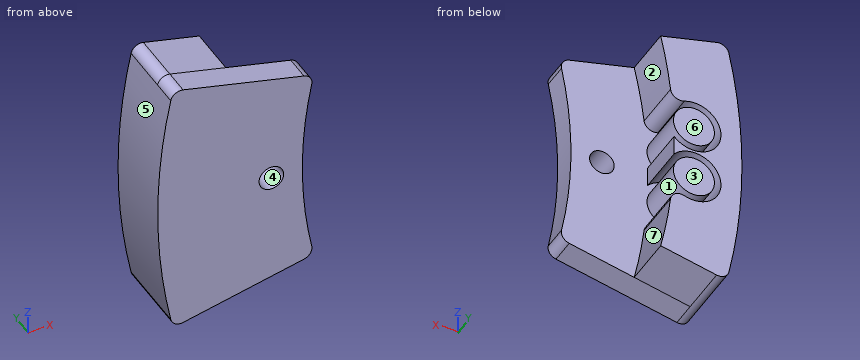
from build123d import *

# Parameters (mm, degrees)
SKETCH2_R           = 2.4
BOSS_EXTRUDE1_DEPTH = 5
BOSS_EXTRUDE2_DEPTH = 10
SKETCH4_R           = 5.27
SKETCH4_R_2         = 4
CUT_EXTRUDE1_DEPTH  = 10
CUT_EXTRUDE2_DEPTH  = 6
FILLET1_R           = 2


with BuildPart() as part:
    # Sketch2 → Boss-Extrude1 (new body)
    with BuildSketch(Plane(origin=(0, 0, 0), x_dir=(1, 0, 0), z_dir=(0, 1, 0))):
        with BuildLine():
            Line((100.252220984, 12.5), (-12.802476078, 38.600733409))
            ThreePointArc((-12.802476078, 38.600733409), (-15.776279016, 12.5), (-12.802476078, -13.600733409))
            Line((-12.802476078, -13.600733409), (100.252220984, 12.5))
        make_face()
        with Locations((6.397320984, 12.5)):
            Circle(SKETCH2_R, mode=Mode.SUBTRACT)
    extrude(amount=BOSS_EXTRUDE1_DEPTH)

    # Sketch3 → Boss-Extrude2 (add)
    with BuildSketch(Plane(origin=(0, 5, 0), x_dir=(1, 0, 0), z_dir=(0, 1, 0))):
        with BuildLine():
            Line((0.080644919, -10.626430568), (-12.802476078, -13.600733409))
            ThreePointArc((-12.802476078, -13.600733409), (-15.776279016, 12.5), (-12.802476078, 38.600733409))
            Line((-12.802476078, 38.600733409), (0.080644919, 35.626430568))
            ThreePointArc((0.080644919, 35.626430568), (-2.554279016, 12.5), (0.080644919, -10.626430568))
        make_face()
    extrude(amount=BOSS_EXTRUDE2_DEPTH)

    # Sketch4 → Cut-Extrude1 (cut)
    with BuildSketch(Plane(origin=(0, 15, 0), x_dir=(1, 0, 0), z_dir=(0, 1, 0))):
        with Locations((-6.412573781, 7)):
            Circle(SKETCH4_R)
        with Locations((-6.412573781, 7)):
            Circle(SKETCH4_R_2, mode=Mode.SUBTRACT)
    cut_extrude1 = extrude(amount=-CUT_EXTRUDE1_DEPTH, mode=Mode.SUBTRACT)

    # Mirror1: Cut-Extrude1 across plane
    add(cut_extrude1.mirror(Plane.XY.offset(-12.5)), mode=Mode.SUBTRACT)

    # Sketch5 → Cut-Extrude2 (cut, through all)
    with BuildSketch(Plane(origin=(0, 5, 0), x_dir=(1, 0, 0), z_dir=(0, 1, 0))):
        with BuildLine():
            Line((14.696195891, -7.252164753), (100.252220984, 12.5))
            Line((100.252220984, 12.5), (14.696195891, 32.252164753))
            ThreePointArc((14.696195891, 32.252164753), (12.445720984, 12.5), (14.696195891, -7.252164753))
        make_face()
    extrude(amount=-CUT_EXTRUDE2_DEPTH, mode=Mode.SUBTRACT)

    # Fillet1
    fillet1_edges = [part.edges().sort_by_distance(p)[0] for p in [
        (-2.189516169, 10, -3.847432094),
        (-2.189516169, 10, -21.152567906),
        (-12.802476078, 7.5, 13.600733409),
        (14.696195891, 2.5, -32.252164753),
        (-12.802476078, 7.5, -38.600733409),
        (14.696195891, 2.5, 7.252164753),
    ]]
    fillet(fillet1_edges, radius=FILLET1_R)


solid = part.part
Source: CAD feature listing. Evaluate the final solid. Frame: model axes, mm. Face numbers are marked on the shaded views. A direction names the side the tool comes from. Give positions to 0.01 mm unless a question says otherwise; leave off trailing zeros. Write each loop counter-clockwise with the first axis right and the second up, starting at its lowest first coordinate (ties: lowest second). Pieces come first, ordered by that corner, then holes. Notation, with made-up numbers: M 65.5,25.5 L 110.5,25.5 A19 ccw 110.5,30.5 Z; hole C -26.5,28 d10. An arc over 180 degrees is marked long. Return JSON: item names as keys, results as strings. Group by question number.
1) Ray query, L1, parallel to Z at x = -10.5, y = 14; L2, parallel to Z at x = -9.5, y = 9.25; L3, parallel to Z at x = -3, y = 7.75. Return the intervals inside material, ascending.
2) Set-up query: the marked faces 1, 2 and 3. Return all of +Z, -Z, +X, -X, +Y, -Y with unobstructed straight access to the full face (end or side cutting, diameter ignored); none if empty.
3) Cut plane C-C, the plane z = -7.5. Output: boundary loops of the cut face in (x, y).
4) Cut plane D-D, the plane y = 6.25. Give the number of separate pieces and of enclosed holes in the cut face, then the cut area to 3 significant figures.
5) Cut plane B-B, the plane x = 5. Output: boundary loops of the cut face in (y, z).
6) Cut plane A-A, the plane y = 3. Output: boundary loops of the cut face in (x, z), then the cut area to 3 significant figures.
7) Draft query along X for the marked faces 4, 5, 6 and 7. Return one class per face: released by +X, released by -X, zero draft, split by the parting line, or undercut.
8) First-contact query: pin 1 Ø1 at (x, y) = (1.5, 2.5) entering from -Z; pin 2 Ø5 at (y, z) = (5.5, -26) entering from -X; pin 3 Ø2 at (x, z) = (7, -31.5) entering from +Y. Flat tips, straight axial feed; report the tip coordinate or a pass-through.
Data:
{
 "1": {"L1": "z = -38.07 to -21.33, -14.67 to -10.33, -3.67 to 13.07", "L2": "z = -37.84 to -22.27, -20.54 to -15.46, -13.73 to -11.27, -9.54 to -4.46, -2.73 to 12.84", "L3": "z = -36.34 to -22.98, -20.09 to -15.91, -13.98 to -11.02, -9.09 to -4.91, -2.02 to 11.34"},
 "2": {"face 1": "+Y", "face 2": "+X, +Y", "face 3": "+Z, -Z, +X, -X, +Y"},
 "3": {"outline": "M -15.67,0 L 12.59,0 L 12.59,5 L -2.44,5 L -2.44,15 L -10.38,15 L -10.38,5 L -11.66,5 L -11.66,15 L -15.67,15 Z"},
 "4": {"separate pieces": "3", "enclosed holes": "0", "area": "588 mm²"},
 "5": {"outline": "M 0,-34.49 L 5,-34.49 L 5,-14.45 L 0,-14.45 Z; M 0,-10.55 L 5,-10.55 L 5,9.49 L 0,9.49 Z"},
 "6": {"outline": "M -13.24,-36.61 A2 ccw -10.84,-38.15 L 12.77,-32.7 A2 ccw 14.28,-30.34 A87.81 cw 14.28,5.34 A2 ccw 12.77,7.7 L -10.84,13.15 A2 ccw -13.24,11.61 A116.03 ccw Z; hole C 6.4,-12.5 d4.8", "area": "1,280 mm²"},
 "7": {"face 4": "undercut", "face 5": "released by -X", "face 6": "zero draft", "face 7": "released by +X"},
 "8": {"pin 1": "stops at z = -35.41", "pin 2": "stops at x = -15.25", "pin 3": "stops at y = 5"}
}
